from build123d import *

# Parameters (mm, degrees)
EXTRUDE_THIN1_DEPTH = 70


with BuildPart() as part:
    # Sketch1 → Extrude-Thin1 (new, symmetric)
    with BuildSketch(Plane(origin=(0, 0, 0), x_dir=(0, 0, -1), z_dir=(1, 0, 0))):
        with BuildLine():
            ThreePointArc((660, 240.220354616), (347.968383065, 70.742450573), (0, 0))
            Line((0, 0), (-1300, 229.225074921))
            Line((-1300, 229.225074921), (-1294.79055467, 258.769307511))
            Line((-1294.79055467, 258.769307511), (1.826085437, 30.140810225))
            ThreePointArc((1.826085437, 30.140810225), (339.301235488, 99.514508401), (641.938605277, 264.174185638))
            Line((641.938605277, 264.174185638), (660, 240.220354616))
        make_face()
    extrude(amount=EXTRUDE_THIN1_DEPTH, both=True)


solid = part.part
The model under review builds one solid part; all positions refer to its coordinate system, in mm. A direction names the side the tool comes from. Coordinates: 2 decimals unless noted, no trailing zeros. Loops run counter-clockwise (first coordinate to the right, second up) from the corner with the lowest first, then second, coordinate; pieces in that order, holes last. Notation, with made-up numbers: M -13.75,58 L 3.25,58 A28 ccw 3.25,97 Z; hole C 25.25,57 d7. An arc over 180 degrees is marked long. Put each result on its own line as item: value. Start each with the question number.
Q1. Add section B-B (x = -54). Write out the cut boundary in (y, z).
Q2. Add section A-A (y = 94.5). Write out the cut boundary in (x, z).
Q3. Wall thickness on line 1 (Y direction, x = 41, z = 309); line 2 (Y direction, x = -13, z = -149): over which ranges is each line inside the solid? List them lowest first.
Q4. Add section D-D (z = -50). Write out the cut boundary in (x, y).
Q5. Add section C-C (y = 209). Write out the cut boundary in (x, z).
Q6. For faces 1 (the flat face through (-70, 84, 315)), 2 (the cylindrical face through (0.98, 97.86, -334.75)), list the 3-axis set-ups (+Z, -Z, +X, -X, +Y, -Y) from which the entire face can be reached by the end or side of a thin tool; tool diameter is ignored.
Q7. Clearance check with flat-ended pins moving along their axes: pin 1 (6 mm diameter, centred on x = -16, z = -399.5, fed in from -Y); pin 2 (1 mm diameter, centred on x = -1, z = 734, fed in from -Y); pin 3 (6 mm diameter, centred on x = 29.5, z = -392.5, fed in from +Y). State where each tip first meets the part, or that it passes through.
Q8. The part is to be moulded in two halves that separate along Z. For faces 3 (the cylindrical face through (0.98, 72.459, -352.653)), 4 (the flat face through (0.98, 113.008, 640.9)), 5 (the flat face through (0.98, 146.055, 655.559)), say which applies: +Z half, -Z half, draft (parallel to the pull), parting line (faces both ways), or undercut.
Answers:
1. outline: M 0,0 A1200 ccw 240.22,-660 L 264.17,-641.94 A1170 cw 30.14,-1.83 L 258.77,1294.79 L 229.23,1300 Z
2. outline: M -70,-408.14 L 70,-408.14 L 70,-325.31 L -70,-325.31 Z; M -70,363.17 L 70,363.17 L 70,535.94 L -70,535.94 Z
3. line 1: y = 54.49 to 84.95
3. line 2: y = 17.15 to 47.64
4. outline: M -70,3.65 L 70,3.65 L 70,33.79 L -70,33.79 Z
5. outline: M -70,-616.62 L 70,-616.62 L 70,-562.08 L -70,-562.08 Z; M -70,1012.53 L 70,1012.53 L 70,1185.3 L -70,1185.3 Z
6. face 1: +Z, -Z, -X, +Y, -Y
6. face 2: +X, -X, +Y
7. pin 1: stops at y = 89.61
7. pin 2: stops at y = 129.34
7. pin 3: stops at y = 121.72
8. face 3: -Z half
8. face 4: +Z half
8. face 5: undercut
